Could you check a few things on this model? Use its own coordinates, in mm. A direction names the side the tool comes from. Give positions to 0.01 mm unless a question says otherwise; leave off trailing zeros. Loops run counter-clockwise (first coordinate to the right, second up) from the corner with the lowest first, then second, coordinate; pieces in that order, holes last. Notation, with made-up numbers: M 58.5,14 L 105.5,14 A13 ccw 105.5,18 Z; hole C 61,17.5 d7. An arc over 180 degrees is marked long. Answer in a Markdown table with one row per item. Add a question column.
1. Thinking about a two-plate mould opening in X: for faces 4 (the flat face through (-93.6, -0.2, 127)), 5 (the conical face through (-119.613, 0.692, 126.753)), 6 (the flat face through (-30.48, 0, 61)), which applies, released by +X, released by -X, zero draft, split by the parting line, or undercut?
2. If we section it at A-A on z = 65.5: Count the separate pieces of the cut face and the enclosed holes in it, then the cut area to 3 significant figures.
3. Which directions (+Z, -Z, +X, -X, +Y, -Y) give clear straight access to the entire face, cutting with the end or side of a thin tool? Please do faces 1 (the cylindrical face through (-28.952, 7.441, 58.959)), 2 (the cylindrical face through (-28.952, -7.441, 58.959)), 3 (the conical face through (-119.684, -0.695, 86.678)).
4. If we section it at B-B on x = -101.6: List the corners of the cut face in (y, z) for me, then the cut area to 3 significant figures.
5. I need wall thicknesses on line 1 along X through (y, z) = (0, 68.5); line 2 along X through (y, z) = (0, 14); line 3 along Z through (x, y) = (-85, 1.5). Which ranges of each line are inside material? Lowest first, please. Write a range as from..to.
6. I'm going to push flat-ended pins straight in: pin 1 Ø1.5 at (x, z) = (-33, 58.5) entering from +Y; pin 2 Ø12 at (x, y) = (0, 0) entering from +Z; pin 3 Ø9 at (y, z) = (-0.5, 45) entering from -X; pin 4 Ø12 at (y, z) = (-21.5, 48) entering from +X. Where does each tip first touch, or does it pass through?
```python
from build123d import *

# Parameters (mm, degrees)
F0_R      = 22.86
F0_R_2    = 7.62
F1_DEPTH  = 127
F0_R_3    = 25.4
F2_DEPTH  = 101.6
F4_DEPTH  = 8.89
F5_W      = 60.96
F5_H      = 60.96
F6_DEPTH  = 50.8
F7_R      = 5.07999
F8_SIZE   = 5.08
F9_R      = 30.48
F10_DEPTH = 12.7
F11_SIZE  = 5.07999


# Not quite as in the source:
# - a fillet or chamfer is up to 0.001 mm smaller than in the source, because OpenCascade refuses the exact size


with BuildPart() as f1:
    # F0 (on Top) → F1 (new body)
    with BuildSketch(Plane.XY):
        with Locations((-101.6, 0)):
            Circle(F0_R)
        with Locations((-101.6, 0)):
            Circle(F0_R_2, mode=Mode.SUBTRACT)
    extrude(amount=F1_DEPTH)



with BuildPart() as f2:
    # F0 (on Top) → F2 (new body)
    with BuildSketch(Plane.XY):
        Circle(F0_R_3)
        Circle(F0_R_2, mode=Mode.SUBTRACT)
    extrude(amount=F2_DEPTH)


with BuildPart() as f1_1:
    add(f1.part)

    add(f2.part)  # F4 merges F2
    # F3 (on Front) → F4 (join, symmetric)
    with BuildSketch(Plane.XZ):
        with BuildLine():
            Line((-81.28, 127), (-81.28, 0))
            Line((-81.28, 0), (-20.32, 0))
            Line((-20.32, 0), (-20.32, 81.28))
            ThreePointArc((-20.32, 81.28), (-40.0155943211, 108.82076155), (-68.58, 127))
            Line((-68.58, 127), (-81.28, 127))
        make_face()
        with BuildLine():
            ThreePointArc((-68.58, 113.1692568198), (-45.7184650999, 96.5627163287), (-30.48, 72.7674195988))
            Line((-30.48, 72.7674195988), (-30.48, 49.6692568198))
            Line((-30.48, 49.6692568198), (-68.58, 49.6692568198))
            Line((-68.58, 49.6692568198), (-68.58, 113.1692568198))
        make_face(mode=Mode.SUBTRACT)
    extrude(amount=F4_DEPTH, both=True)

    # F5 (on Front) → F6 (cut, symmetric)
    with BuildSketch(Plane.XZ):
        with Locations((-104.14, 55.88)):
            Rectangle(F5_W, F5_H)
    extrude(amount=F6_DEPTH, both=True, mode=Mode.SUBTRACT)

    # F7 (radius 5.08 in the source; OpenCascade refuses exactly that, so slightly less here)
    f7_edges = [f1_1.edges().sort_by_distance(p)[0] for p in [
        (-45.718465, -8.89, 96.562716),
        (-30.48, -8.89, 61.218338),
        (-49.53, -8.89, 49.669257),
        (-68.58, -8.89, 81.419257),
        (-45.718465, 8.89, 96.562716),
        (-30.48, 8.89, 61.218338),
        (-49.53, 8.89, 49.669257),
        (-68.58, 8.89, 81.419257),
    ]]
    fillet(f7_edges, radius=F7_R)

    # F8
    f8_edges = [f1_1.edges().sort_by_distance(p)[0] for p in [
        (-124.46, 0, 86.36),
        (-124.46, 0, 0),
        (-124.46, 0, 25.4),
        (-124.46, 0, 127),
    ]]
    chamfer(f8_edges, length=F8_SIZE)

    # F9 (on Top) → F10 (join)
    with BuildSketch(Plane.XY):
        Circle(F9_R)
        with BuildLine():
            Line((-62.23, 2.54), (-62.23, -2.54))
            Line((-62.23, -2.54), (-31.6482369177, -2.54))
            ThreePointArc((-31.6482369177, -2.54), (-31.75, 0), (-31.6482369177, 2.54))
            Line((-31.6482369177, 2.54), (-62.23, 2.54))
        make_face()
    extrude(amount=F10_DEPTH)

    # F11 (size 5.08 in the source; OpenCascade refuses exactly that, so slightly less here)
    f11_edges = [f1_1.edges().sort_by_distance(p)[0] for p in [
        (30.48, 0, 12.7),
        (-25.4, 0, 101.6),
        (-7.62, 0, 101.6),
    ]]
    chamfer(f11_edges, length=F11_SIZE)


solid = f1_1.part
```
Results:
| question | item | result |
|---|---|---|
| 1 | face 4 | zero draft |
| 1 | face 5 | split by the parting line |
| 1 | face 6 | undercut |
| 2 | separate pieces | 2 |
| 2 | enclosed holes | 1 |
| 2 | area | 2,010 mm2 |
| 3 | face 1 | +Y |
| 3 | face 2 | -Y |
| 3 | face 3 | none |
| 4 | outline | M -22.86,5.08 L -17.78,0 L -7.62,0 L -7.62,25.4 L -17.78,25.4 L -22.86,20.32 Z; M -22.86,91.44 L -17.78,86.36 L -7.62,86.36 L -7.62,127 L -17.78,127 L -22.86,121.92 Z; M 7.62,0 L 17.78,0 L 22.86,5.08 L 22.86,20.32 L 17.78,25.4 L 7.62,25.4 Z; M 7.62,86.36 L 17.78,86.36 L 22.86,91.44 L 22.86,121.92 L 17.78,127 L 7.62,127 Z |
| 4 | area | 1,910 mm2 |
| 5 | line 1 | -73.66..-68.58, -30.48..-7.62, 7.62..25.4 |
| 5 | line 2 | -124.46..-109.22, -93.98..-7.62, 7.62..25.4 |
| 5 | line 3 | 0..25.4, 86.36..127 |
| 6 | pin 1 | through |
| 6 | pin 2 | z = 12.7 |
| 6 | pin 3 | x = -73.66 |
| 6 | pin 4 | x = 20.12 |
